Here's how the part is built. I have some questions about the finished solid (model axes, mm). A direction names the side the tool comes from. Give positions to 0.01 mm unless a question says otherwise; leave off trailing zeros. Order: outer loops, then holes, each group sorted by start corner. A loop starts at its lowest first (then second) coordinate and runs counter-clockwise, first axis right, second up.
from build123d import *

# Parameters (mm, degrees)
SKETCH_1_W          = 20
SKETCH_1_H          = 20
EXTRUDE_1_DEPTH     = 60
SKETCH_7_W          = 26
SKETCH_7_H          = 6
CUT_EXTRUDE_6_DEPTH = 34
SKETCH_2_R          = 6.5
CUT_EXTRUDE_9_DEPTH = 5
SKETCH_3_R          = 4.5
CUT_EXTRUDE_2_DEPTH = 29
MOVE_BODY_1_ANGLE   = 90
SKETCH_8_W          = 20
SKETCH_8_H          = 20
EXTRUDE_2_DEPTH     = 8
FILLET_2_R          = 7


# Read off the part's stored shape, not the designer's step: the other step
with BuildPart() as part:
    # Sketch 1 → Extrude 1 (new body)
    with BuildSketch(Plane.XY):
        Rectangle(SKETCH_1_W, SKETCH_1_H)
    extrude(amount=EXTRUDE_1_DEPTH)

    # Sketch 7 → Cut-Extrude 6 (cut)
    with BuildSketch(Plane(origin=(10, 0, 0), x_dir=(0, 0, -1), z_dir=(1, 0, 0))):
        with Locations((-13, 7)):
            Rectangle(SKETCH_7_W, SKETCH_7_H)
        with Locations((-13, -7)):
            Rectangle(SKETCH_7_W, SKETCH_7_H)
    cut_extrude_6 = extrude(amount=-CUT_EXTRUDE_6_DEPTH, mode=Mode.SUBTRACT)

    # Sketch 2 → Cut-Extrude 9 (cut)
    with BuildSketch(Plane(origin=(0, 4, 0), x_dir=(-1, 0, 0), z_dir=(0, -1, 0))):
        with Locations(Location((0, -10.902706153, 0), (0, 0, 90))):
            Circle(SKETCH_2_R)
    cut_extrude_9 = extrude(amount=CUT_EXTRUDE_9_DEPTH, mode=Mode.SUBTRACT)

    # Sketch 3 → Cut-Extrude 2 (cut)
    with BuildSketch(Plane(origin=(0, -4, 0), x_dir=(-1, 0, 0), z_dir=(0, -1, 0))):
        with Locations(Location((0, -10.902706153, 0), (0, 0, 90))):
            Circle(SKETCH_3_R)
        with BuildLine():
            Line((-21.262122506, -10.902706153), (-10, -10.902706153))
            ThreePointArc((-10, -10.902706153), (0, -0.902706153), (10, -10.902706153))
            Line((10, -10.902706153), (21.262122506, -10.902706153))
            ThreePointArc((21.262122506, -10.902706153), (0, 10.359416353), (-21.262122506, -10.902706153))
        make_face()
    cut_extrude_2 = extrude(amount=-CUT_EXTRUDE_2_DEPTH, mode=Mode.SUBTRACT)

    # Mirror 6: Cut-Extrude 6, Cut-Extrude 9, Cut-Extrude 2 across plane
    add(cut_extrude_6.mirror(Plane.XY.offset(30)), mode=Mode.SUBTRACT)
    add(cut_extrude_9.mirror(Plane.XY.offset(30)), mode=Mode.SUBTRACT)
    add(cut_extrude_2.mirror(Plane.XY.offset(30)), mode=Mode.SUBTRACT)


with BuildPart() as body_2:
    # Other 3: the piece on the far side of the plane
    add(part.part)
    split(bisect_by=Plane.XY.offset(30), keep=Keep.BOTTOM)


with BuildPart() as part_1:
    add(part.part)

    # Other 3
    split(bisect_by=Plane.XY.offset(30), keep=Keep.TOP)


with BuildPart() as part_2:
    # Move Body 1: moved
    add(part_1.part.rotate(Axis((0, 0, 0), (0, 0, 1)), MOVE_BODY_1_ANGLE))


    add(body_2.part)  # Extrude 2 merges body 2
    # Sketch 8 → Extrude 2 (add)
    with BuildSketch(Plane.XY.offset(34)):
        Rectangle(SKETCH_8_W, SKETCH_8_H)
    extrude(amount=-EXTRUDE_2_DEPTH)

    # Fillet 2
    # the kernel refuses this fillet: 7 mm, written as the material it adds along each edge
    with BuildSketch(Plane(origin=(-4, 10, 34), x_dir=(0, 0, 1), z_dir=(0, -1, 0)), Plane(origin=(10, -4, 26), x_dir=(0, 0, -1), z_dir=(-1, 0, 0))) as fillet_2_piece_1:
        with BuildLine():
            CenterArc((6.92820323, 7), FILLET_2_R, 188.213210702, 81.786789298)
            Line((0, 6), (-0.138564065, 5.98))
            ThreePointArc((-0.138564065, 5.98), (-0.14, 3), (-0.14, 0))
            Line((-0.14, 0), (0, -0.14))
            Line((0, -0.14), (6.92820323, -0.14))
            Line((6.92820323, -0.14), (6.92820323, 0))
        make_face()
    extrude(amount=20)
    with BuildSketch(Plane(origin=(4, 10, 34), x_dir=(1, 0, 0), z_dir=(0, -1, 0))) as fillet_2_piece_2:
        with BuildLine():
            CenterArc((7, 6.92820323), FILLET_2_R, 180, 81.786789298)
            Line((0, 6.92820323), (-0.14, 6.92820323))
            Line((-0.14, 6.92820323), (-0.14, 0))
            Line((-0.14, 0), (0, -0.14))
            ThreePointArc((0, -0.14), (3, -0.14), (5.98, -0.138564065))
            Line((5.98, -0.138564065), (6, 0))
        make_face()
    extrude(amount=20)
    with BuildSketch(Plane(origin=(10, 4, 26), x_dir=(0, 0, -1), z_dir=(-1, 0, 0))) as fillet_2_piece_3:
        with BuildLine():
            CenterArc((6.92820323, -7), FILLET_2_R, 90, 81.786789298)
            Line((0, -6), (-0.138564065, -5.98))
            ThreePointArc((-0.138564065, -5.98), (-0.14, -3), (-0.14, 0))
            Line((-0.14, 0), (0, 0.14))
            Line((0, 0.14), (6.92820323, 0.14))
            Line((6.92820323, 0.14), (6.92820323, 0))
        make_face()
    extrude(amount=20)


solid = part_2.part
Q1. Thinking about a two-plate mould opening in Z: for faces 1 (the face through (-4, 5, 54)), 2 (the face through (1, 4.42, 47.56)), 3 (the face through (0.14, -5.755, 23.707)), 4 (the face through (1.35, -2.52, 6.61)), which applies, released by +Z, released by -Z, zero draft, split by the parting line, or undercut?
Filled sheet:
face 1: zero draft
face 2: undercut
face 3: released by -Z
face 4: undercut
Q2. If we section it at A-A on x = 0: List the corners of the cut face in (y, z) for me, plus the area to 3 significant figures.
Filled sheet:
outline: (-10, 26) arc R7 cw to (-4, 19.07) - (-4, 15.4) - (-1, 15.4) - (-1, 17.4) - (4, 17.4) - (4, 19.07) arc R7 cw to (10, 26) - (10, 49.1) arc R10 ccw to (-10, 49.1) - close; (-4, 0.9) - (4, 0.9) - (4, 4.4) - (-1, 4.4) - (-1, 6.4) - (-4, 6.4) - close; hole circle Ø13 at (0, 49.1)
area: 615 mm2
Q3. I need wall thicknesses on L1, parallel to X at y = 1, z = 11; L2, parallel to Z at x = 1.25, y = 0; L3, parallel to Z at x = 2.3, y = 0. Which ranges of each line are inside material? Lowest first, please.
Filled sheet:
L1: x = -10 to -6.5, 6.5 to 10
L2: z = 0.98 to 4.52, 17.28 to 44.6, 53.6 to 59.1
L3: z = 1.17 to 4.82, 16.98 to 44.6, 53.6 to 59.1
Q4. If we section it at C-C on y = -7.75: List the corners of the cut face in (x, z) for me.
Filled sheet:
outline: (-10, 25.27) - (10, 25.27) - (10, 34) arc R7 cw to (4, 40.93) - (4, 55.42) - (-4, 55.42) - (-4, 40.93) arc R7 cw to (-10, 34) - close
Q5. If we section it at B-B on y = 0: List the corners of the cut face in (x, z) for me, plus the area to 3 significant figures.
Filled sheet:
outline: (-10, 10.9) arc R10 ccw to (10, 10.9) - (10, 34) arc R7 cw to (4, 40.93) - (4, 44.6) - (1, 44.6) - (1, 42.6) - (-4, 42.6) - (-4, 40.93) arc R7 cw to (-10, 34) - close; (-4, 55.6) - (1, 55.6) - (1, 53.6) - (4, 53.6) - (4, 59.1) - (-4, 59.1) - close; hole circle Ø13 at (0, 10.9)
area: 615 mm2
Q6. For faces 5 (the face through (5, -4, 10)), 6 (the face through (-3.955, 1.535, 16.061)), 7 (the face through (5, 4, 6)), which set-ups out of +Z, -Z, +X, -X, +Y, -Y let a thin tool reach every point of the face, with its end or its side?
Filled sheet:
face 5: -Z, +X, -X, -Y
face 6: +Y
face 7: -Z, +X, -X, +Y
Q7. I'm going to push flat-ended pins straight in: P1, Ø11.5, axis at x = 0, z = 10.9, coming from the -Y side; P2, Ø12, axis at x = -0.5, z = 17, coming from the -Y side; P3, Ø10.5, axis at y = 1.5, z = 47.5, coming from the -X side; P4, Ø7, axis at x = 0, z = 10.9, coming from the +Y side. Where does each tip first touch, or does it pass through?
Filled sheet:
P1: stops at y = -4
P2: stops at y = -5.21
P3: stops at x = -4
P4: passes through
